Input: part model. Units: mm. Frame: model coordinates. Round coordinates to 2 decimals unless told otherwise and drop trailing zeros. Loops run counter-clockwise (first coordinate to the right, second up) from the corner with the lowest first, then second, coordinate; pieces in that order, holes last.
(1) Line query: line 1 (Z direction, x = -2, y = -11.25); line 2 (X direction, y = -1, z = 343.5); line 3 (X direction, y = -3.5, z = 19.5). Output: solid intervals per line, ascending.
(2) Cut plane B-B, the plane z = 62. Output: boundary loops of the cut face in (x, y).
(3) First-contact query: pin 1 Ø3.5 at (x, y) = (-5.5, -7.5) entering from -Z; pin 2 Ø3.5 at (y, z) = (-8, 15) entering from -X; pin 3 Ø6 at (x, y) = (87.5, -1.5) entering from -Z; pin 4 Ø10 at (x, z) = (100.5, 198.5) entering from +Y. Flat tips, straight axial feed; report the tip coordinate or a pass-through.
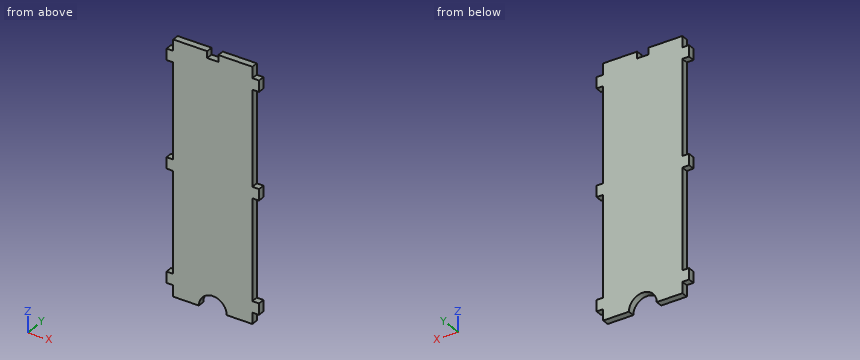
from build123d import *

# Parameters (mm, degrees)
F0_W      = 142.05
F0_H      = 460
F1_DEPTH  = 12
F2_W      = 10
F2_H      = 20
F3_DEPTH  = 12
F4_DEPTH  = 25
F5_DEPTH  = 2
F7_DEPTH  = 25
F8_DEPTH  = 10
F9_DEPTH  = 2
F10_DEPTH = 2


with BuildPart() as f1:
    # F0 (on Front) → F1 (new body)
    with BuildSketch(Plane.XZ):
        with Locations((71.025, 230)):
            Rectangle(F0_W, F0_H)
    extrude(amount=F1_DEPTH)

    # F2 (on face) → F3 (join)
    with BuildSketch(Plane.XZ.offset(12)):
        with Locations((-5, 420)):
            Rectangle(F2_W, F2_H)
        with Locations((147.05, 420)):
            Rectangle(F2_W, F2_H)
        with Locations((-5, 230)):
            Rectangle(F2_W, F2_H)
        with Locations((147.05, 230)):
            Rectangle(F2_W, F2_H)
        with Locations((-5, 30)):
            Rectangle(F2_W, F2_H)
        with Locations((147.05, 30)):
            Rectangle(F2_W, F2_H)
    extrude(amount=-F3_DEPTH)

    # F2 (on face) → F4 (cut)
    with BuildSketch(Plane.XZ.offset(12)):
        Polygon((61.025, 480), (61.025, 460), (71.025, 460), (81.025, 460), (81.025, 480), align=None)
        Polygon((71.025, 460), (61.025, 460), (61.025, 440), (81.025, 440), (81.025, 460), align=None)
    extrude(amount=-F4_DEPTH, mode=Mode.SUBTRACT)

    # F5 (cut): a face of the model
    f5_faces = [f1.faces().sort_by_distance(p)[0] for p in [
        (71.025, -6, 440),
    ]]
    extrude(f5_faces, amount=-F5_DEPTH, mode=Mode.SUBTRACT)

    # F6 (on face) → F7 (cut)
    with BuildSketch(Plane.XZ.offset(12)):
        with BuildLine():
            Line((46.025, 0), (96.025, 0))
            ThreePointArc((96.025, 0), (71.025, 25), (46.025, 0))
        make_face()
    extrude(amount=-F7_DEPTH, mode=Mode.SUBTRACT)

    # F8 (cut): faces of the model
    f8_faces = [f1.faces().sort_by_distance(p)[0] for p in [
        (30.5125, -6, 460),
        (111.5375, -6, 460),
    ]]
    extrude(f8_faces, amount=-F8_DEPTH, mode=Mode.SUBTRACT)

    # F9 (add): faces of the model
    f9_faces = [f1.faces().sort_by_distance(p)[0] for p in [
        (152.05, -6, 420),
        (152.05, -6, 230),
        (152.05, -6, 30),
    ]]
    extrude(f9_faces, amount=F9_DEPTH)

    # F10 (add): faces of the model
    f10_faces = [f1.faces().sort_by_distance(p)[0] for p in [
        (-10, -6, 420),
        (-10, -6, 230),
        (-10, -6, 30),
    ]]
    extrude(f10_faces, amount=F10_DEPTH)


solid = f1.part
Reported:
1. line 1: z = 20 to 40, 220 to 240, 410 to 430
1. line 2: x = 0 to 142.05
1. line 3: x = 0 to 55.38, 86.67 to 142.05
2. outline: (0, -12) - (142.05, -12) - (142.05, 0) - (0, 0) - close
3. pin 1: stops at z = 20
3. pin 2: stops at x = 0
3. pin 3: stops at z = 15.68
3. pin 4: stops at y = 0
